from build123d import *

# Parameters (mm, degrees)
F1_DEPTH      = 32.5
F2_R          = 3.7508720601
F3_DEPTH      = 35
F3_DEPTH_BACK = 50
F4_R          = 4.8477507868
F5_DEPTH      = 63.4
F6_R          = 3.4336134654
F7_DEPTH      = 90


with BuildPart() as f1:
    # F0 (on Front) → F1 (new body, symmetric)
    with BuildSketch(Plane.XZ):
        Polygon((3.7480990784, -6.5026984116), (7.5055515568, -0.005400188), (3.7574524784, 6.4972982236), (-3.7480990784, 6.5026984116), (-7.5055515568, 0.005400188), (-3.7574524784, -6.4972982236), align=None)
    extrude(amount=F1_DEPTH, both=True)

    # F2 (on face) → F3 (join, two sides)
    with BuildSketch(Plane(origin=(0.0046767, 0, 6.4999983176), x_dir=(0.9999997412, 0, -0.0007194923), z_dir=(0.0007194923, 0, 0.9999997412))) as f3_sk:
        with Locations((0, 21.6074604541)):
            Circle(F2_R)
    extrude(amount=F3_DEPTH)
    extrude(f3_sk.sketch, amount=-F3_DEPTH_BACK)

    # F4 (on face) → F5 (cut)
    with BuildSketch(Plane.XZ.offset(32.5)):
        Circle(F4_R)
    extrude(amount=-F5_DEPTH, mode=Mode.SUBTRACT)

    # F6 (on face) → F7 (cut)
    with BuildSketch(Plane(origin=(0, 32.5, 0), x_dir=(-1, 0, 0), z_dir=(0, 1, 0))):
        Circle(F6_R)
    extrude(amount=-F7_DEPTH, mode=Mode.SUBTRACT)


solid = f1.part
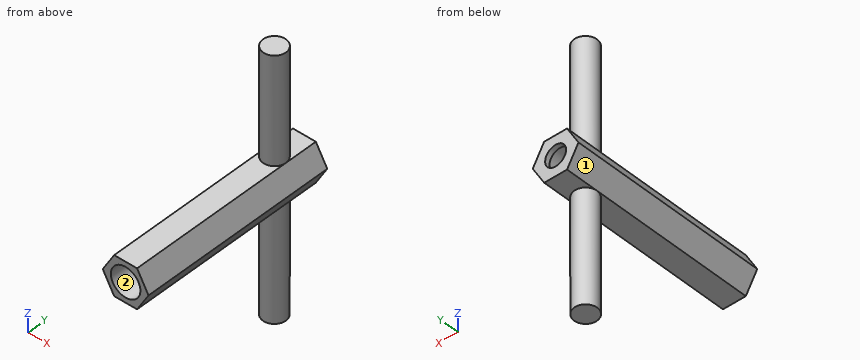
Here's how the part is built. I have some questions about the finished solid (model axes, mm). Face numbers are marked on the shaded views. Give positions to 0.01 mm unless a question says otherwise; leave off trailing zeros. Order: outer loops, then holes, each group sorted by start corner. A loop starts at its lowest first (then second) coordinate and runs counter-clockwise, first axis right, second up. Notation, with made-up numbers: (32.5, 39) -> (38.5, 39) arc R27 ccw to (38.5, 68) -> close; hole circle Ø5 at (68, 5.5). An arc over 180 degrees is marked (long way). Use a Markdown table: item, result. Add a question column.
Item 1: Will these pins go through, and if not, where does the flat tip stop? pin 1 (5 mm diameter, centred on x = -0.5, z = -1, fed in from -Y); pin 2 (1.5 mm diameter, centred on x = -3, y = 16.5, fed in from -Z); pin 3 (4 mm diameter, centred on x = 5, z = -10.5, fed in from -Y).
Item 2: I need wall thicknesses on line 1 (Z direction, x = -0.25, y = 10); line 2 (Z direction, x = 0, y = 31.55); line 3 (Y direction, x = 4, z = -0.5). Which ranges of each line are inside material? Lowest first, please.
Item 3: If we mould it in two halves opening along Z, with no side actions, what happens to the marked faces 1 and 2? For each: pulls with the +Z half, pulls with the -Z half, needs draft (parallel to the pull), parting line crosses it, or undercut.
Item 4: Imagine slicing it at A-A on y = -19. Please give me the cut outline in (x, z).
Data:
| question | item | result |
|---|---|---|
| 1 | pin 1 | stops at y = 30.9 |
| 1 | pin 2 | stops at z = -6.5 |
| 1 | pin 3 | stops at y = 19.37 |
| 2 | line 1 | z = -6.5 to -4.84, 4.84 to 6.5 |
| 2 | line 2 | z = -6.5 to -3.43, 3.43 to 6.5 |
| 2 | line 3 | y = 30.9 to 32.5 |
| 3 | face 1 | pulls with the -Z half |
| 3 | face 2 | undercut |
| 4 | outline | (-7.51, 0.01) -> (-3.76, -6.5) -> (3.75, -6.5) -> (7.51, -0.01) -> (3.76, 6.5) -> (-3.75, 6.5) -> close; hole circle Ø9.7 at (0, 0) |
